Drawing for the job (mm, zero at the part's lowest x, y, z). A direction names the side the tool comes from. Give positions to 0.01 mm unless a question says otherwise; leave off trailing zeros. Loops run counter-clockwise (first coordinate to the right, second up) from the corner with the lowest first, then second, coordinate; pieces in that order, holes last. Notation, with made-up numbers: M -8.5,-11.5 L 50.5,-11.5 A16 ccw 50.5,15.5 Z; hole C 22.25,87 d1. An arc over 180 degrees is marked long. Use CSV: the item, a comma, the result in double quotes. Start each with the question number.
(1) Flat gauge pin, fed straight in: P1, Ø1.5, axis at x = 10.5, z = 11, coming from the +Y side (3 decimals). Where does the tip first touch, or does it go through?
(2) Slice it at D-D on x = 18.25. List the corners of the cut face in (y, z) (3 decimals), and give its area (3 significant figures).
(3) Tool access for the marked faces 5 and 6: list every direction of +Z, -Z, +X, -X, +Y, -Y with a clear straight run to the whole face (end or side of a thin tool).
(4) Wall check: line 1 along Z through (x, y) = (24.13, 7.25) (3 decimals); line 2 along X through (y, z) = (3.25, 17.75); line 3 along Z through (x, y) = (2, 8.25). Give the ranges that are in metal, low to high. Write a range as from..to.
(5) Slice it at B-B on z = 2.54. List the corners of the cut face in (x, y) (3 decimals), and give its area (3 significant figures).
(6) Slice it at C-C on x = 2.54. List the corners of the cut face in (y, z) (3 decimals), and give its area (3 significant figures).
(7) Two-plate mould, pull along Z, no slides. Class the marked faces 1, 2, 3 and 4: pulls with the +Z half, pulls with the -Z half, needs draft (parallel to the pull), parting line crosses it, or undercut.
(8) Slice it at A-A on y = 6. List the corners of the cut face in (x, z) (3 decimals), and give its area (3 significant figures).
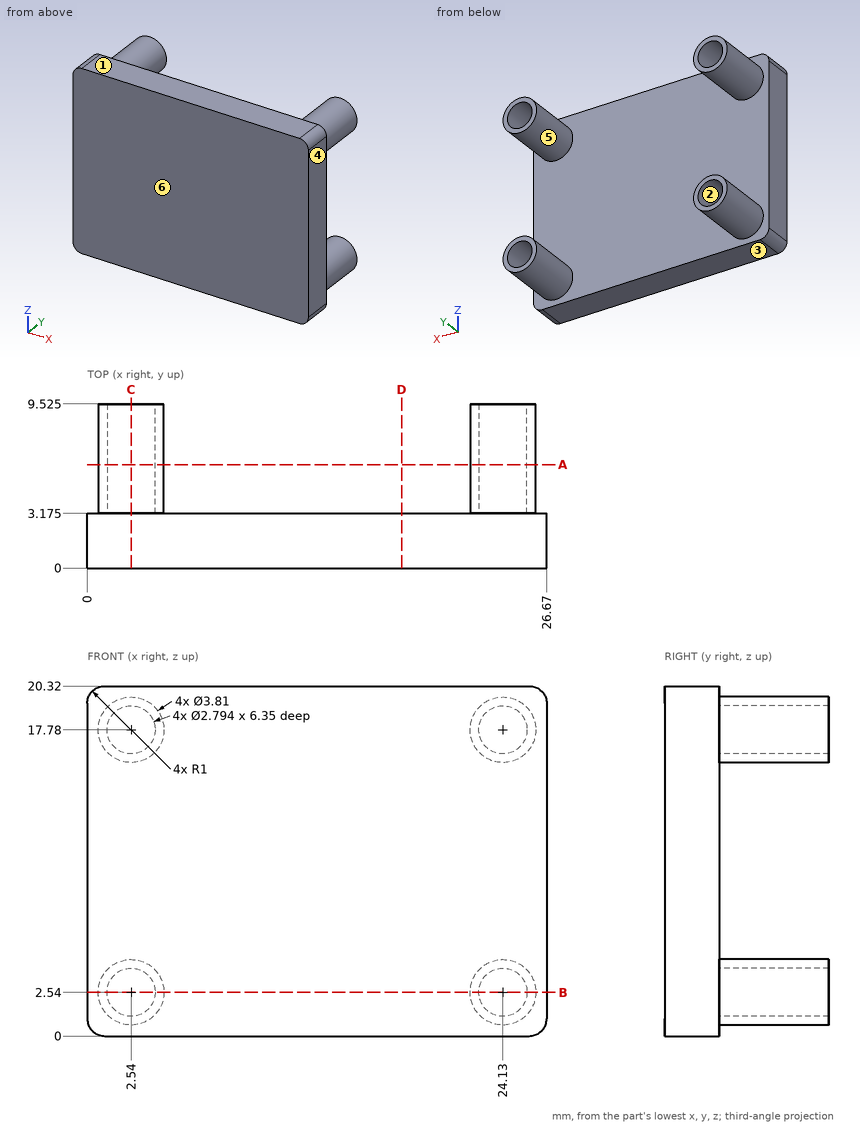
Reply:
1,P1,"stops at y = 3.175"
2,outline,"M 0,0 L 3.175,0 L 3.175,20.32 L 0,20.32 Z"
2,area,"64.5 mm^2"
3,face 5,"+Y"
3,face 6,"+Z, -Z, +X, -X, -Y"
4,line 1,"z = 0.635..1.143, 3.937..4.445, 15.875..16.383, 19.177..19.685"
4,line 2,"x = 0.64..1.14, 3.94..4.44, 22.23..22.73, 25.53..26.03"
4,line 3,"z = 0.71..1.25, 3.83..4.37, 15.95..16.49, 19.07..19.61"
5,outline,"M 0,0 L 26.67,0 L 26.67,3.175 L 26.035,3.175 L 26.035,9.525 L 25.527,9.525 L 25.527,3.175 L 22.733,3.175 L 22.733,9.525 L 22.225,9.525 L 22.225,3.175 L 4.445,3.175 L 4.445,9.525 L 3.937,9.525 L 3.937,3.175 L 1.143,3.175 L 1.143,9.525 L 0.635,9.525 L 0.635,3.175 L 0,3.175 Z"
5,area,"97.6 mm^2"
6,outline,"M 0,0 L 3.175,0 L 3.175,0.635 L 9.525,0.635 L 9.525,1.143 L 3.175,1.143 L 3.175,3.937 L 9.525,3.937 L 9.525,4.445 L 3.175,4.445 L 3.175,15.875 L 9.525,15.875 L 9.525,16.383 L 3.175,16.383 L 3.175,19.177 L 9.525,19.177 L 9.525,19.685 L 3.175,19.685 L 3.175,20.32 L 0,20.32 Z"
6,area,"77.4 mm^2"
7,face 1,"pulls with the +Z half"
7,face 2,"undercut"
7,face 3,"pulls with the -Z half"
7,face 4,"needs draft"
8,outline,"C 2.54,2.54 d3.81; C 2.54,17.78 d3.81; C 24.13,2.54 d3.81; C 24.13,17.78 d3.81; hole C 2.54,2.54 d2.794; hole C 2.54,17.78 d2.794; hole C 24.13,2.54 d2.794; hole C 24.13,17.78 d2.794"
8,area,"21.1 mm^2"
